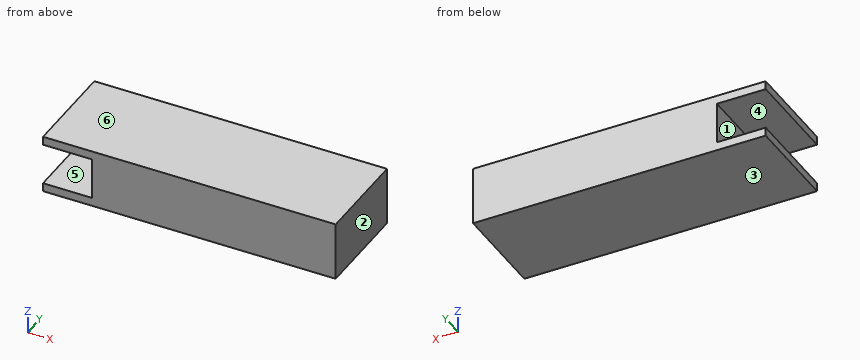
from build123d import *

# Parameters (mm, degrees)
SKETCH1_W           = 30
SKETCH1_H           = 6
BOSS_EXTRUDE1_DEPTH = 10
SKETCH1_4_W         = 5
SKETCH1_4_H         = 4.25
CUT_EXTRUDE1_DEPTH  = 31.822070015


with BuildPart() as part:
    # Sketch1 → Boss-Extrude1 (new body)
    with BuildSketch(Plane(origin=(0, 0, 0), x_dir=(1, 0, 0), z_dir=(0, 1, 0))):
        with Locations((14, 0)):
            Rectangle(SKETCH1_W, SKETCH1_H)
    extrude(amount=BOSS_EXTRUDE1_DEPTH)

    # Sketch1<4> → Cut-Extrude1 (cut, through all)
    with BuildSketch(Plane(origin=(0, 0, 0), x_dir=(1, 0, 0), z_dir=(0, 1, 0))):
        with Locations((1.5, 0)):
            Rectangle(SKETCH1_4_W, SKETCH1_4_H)
    extrude(amount=CUT_EXTRUDE1_DEPTH, mode=Mode.SUBTRACT)


solid = part.part
Can you work these out from the model? Positions are in its coordinate system, mm. Face numbers are marked on the shaded views. A direction names the side the tool comes from. Coordinates: 2 decimals unless noted, no trailing zeros. Write each loop counter-clockwise with the first axis right and the second up, starting at its lowest first coordinate (ties: lowest second). Pieces come first, ordered by that corner, then holes. Notation, with made-up numbers: (79.25, 74.25) -> (128.25, 74.25) arc R15 cw to (128.25, 102.25) -> close; hole circle Ø5 at (82.25, 36.25). An arc over 180 degrees is marked (long way). Write each question's results on one line, items separated by ' | '. Start each with the question number.
Q1. I'm going to push a flat-ended pin straight in: pin 1 (1 mm diameter, centred on y = 6.5, z = -1.5, fed in from -X). Where does the tip first touch, or does it pass through?
Q2. If I drill on probe 1 along Z at (x, y) = (1.75, 4.5) (3 decimals); probe 2 along X at (y, z) = (0.5, -0.2), over which ranges is the centre line in solid material (lowest first)?
Q3. Imagine slicing it at A-A (x = 1.75). Write out the boundary of the cut face in (y, z) (3 decimals), then the cut area to 3 significant figures.
Q4. Imagine slicing it at C-C (z = 0.35). Write out the boundary of the cut face in (x, y).
Q5. Imagine slicing it at B-B (y = 6.25). Write out the boundary of the cut face in (x, z) (3 decimals).
Q6. On a 3-axis mill with a long thin cutter (end or side, diameter ignored), from which of +Z, -Z, +X, -X, +Y, -Y can I reach the whole of each face in a straight line? I mean the marked faces 5 and 6. Say none if no direction works.
Q7. We'd pull the mould along Z, two halves only. Please class the marked faces 1, 2, 3 and 4: +Z half, -Z half, draft (parallel to the pull), parting line (faces both ways), or undercut.
Taken from the geometry:
1) pin 1: stops at x = 4
2) probe 1: z = -3 to -2.125, 2.125 to 3 | probe 2: x = 4 to 29
3) outline: (0, -3) -> (10, -3) -> (10, -2.125) -> (0, -2.125) -> close; (0, 2.125) -> (10, 2.125) -> (10, 3) -> (0, 3) -> close | area: 17.5 mm^2
4) outline: (4, 0) -> (29, 0) -> (29, 10) -> (4, 10) -> close
5) outline: (-1, -3) -> (29, -3) -> (29, 3) -> (-1, 3) -> (-1, 2.125) -> (4, 2.125) -> (4, -2.125) -> (-1, -2.125) -> close
6) face 5: -X, +Y, -Y | face 6: +Z, +X, -X, +Y, -Y
7) face 1: undercut | face 2: draft | face 3: -Z half | face 4: undercut
